Geometry check sheet. Reference: the model listing, model coordinates, mm. A direction names the side the tool comes from. Coordinates: 2 decimals unless noted, no trailing zeros. Write each loop counter-clockwise with the first axis right and the second up, starting at its lowest first coordinate (ties: lowest second). Pieces come first, ordered by that corner, then holes.
from build123d import *

# Parameters (mm, degrees)
SKETCH3_W           = 38.1
SKETCH3_H           = 38.1
BOSS_EXTRUDE2_DEPTH = 1.524
SKETCH4_W           = 16.002
SKETCH4_H           = 16.002
BOSS_EXTRUDE3_DEPTH = 7.112
SKETCH5_R           = 7.493
BOSS_EXTRUDE4_DEPTH = 12.192
BOSS_EXTRUDE6_DEPTH = 7.112


with BuildPart() as part:
    # Sketch3 → Boss-Extrude2 (new body)
    with BuildSketch(Plane(origin=(0, 0, 0), x_dir=(1, 0, 0), z_dir=(0, 1, 0))):
        Rectangle(SKETCH3_W, SKETCH3_H)
    extrude(amount=BOSS_EXTRUDE2_DEPTH)

    # Sketch4 → Boss-Extrude3 (add)
    with BuildSketch(Plane(origin=(0, 1.524, 0), x_dir=(1, 0, 0), z_dir=(0, 1, 0))):
        Rectangle(SKETCH4_W, SKETCH4_H)
    extrude(amount=BOSS_EXTRUDE3_DEPTH)

    # Sketch5 → Boss-Extrude4 (add)
    with BuildSketch(Plane(origin=(0, 8.636, 0), x_dir=(1, 0, 0), z_dir=(0, 1, 0))):
        with Locations(Location((0, 0, 0), (0, 0, 90))):
            Circle(SKETCH5_R)
    extrude(amount=BOSS_EXTRUDE4_DEPTH)

    # Sketch6 → Boss-Extrude6 (add)
    with BuildSketch(Plane(origin=(0, 8.636, 0), x_dir=(1, 0, 0), z_dir=(0, 1, 0))):
        with BuildLine():
            ThreePointArc((8.001, -0.71842049), (8.768319307, -1.717057132), (9.9695, -2.0955))
            ThreePointArc((9.9695, -2.0955), (11.45124226, -1.48174226), (12.065, 0))
            ThreePointArc((12.065, 0), (11.45124226, 1.48174226), (9.9695, 2.0955))
            ThreePointArc((9.9695, 2.0955), (8.768319307, 1.717057132), (8.001, 0.71842049))
            Line((8.001, 0.71842049), (8.001, -0.71842049))
        make_face()
        with BuildLine():
            ThreePointArc((8.001, 0.71842049), (7.874, 0), (8.001, -0.71842049))
            Line((8.001, -0.71842049), (8.001, 0.71842049))
        make_face()
        with BuildLine():
            Line((8.001, -2.0955), (9.9695, -2.0955))
            ThreePointArc((9.9695, -2.0955), (8.768319307, -1.717057132), (8.001, -0.71842049))
            Line((8.001, -0.71842049), (8.001, -2.0955))
        make_face()
        with BuildLine():
            Line((7.194020347, -2.0955), (8.001, -2.0955))
            Line((8.001, -2.0955), (8.001, -0.71842049))
            ThreePointArc((8.001, -0.71842049), (7.874, 0), (8.001, 0.71842049))
            Line((8.001, 0.71842049), (8.001, 2.0955))
            Line((8.001, 2.0955), (7.194020347, 2.0955))
            ThreePointArc((7.194020347, 2.0955), (7.417878519, 1.058360652), (7.493, 0))
            ThreePointArc((7.493, 0), (7.417878519, -1.058360652), (7.194020347, -2.0955))
        make_face()
        with BuildLine():
            ThreePointArc((8.001, 0.71842049), (8.768319307, 1.717057132), (9.9695, 2.0955))
            Line((9.9695, 2.0955), (8.001, 2.0955))
            Line((8.001, 2.0955), (8.001, 0.71842049))
        make_face()
        with BuildLine():
            Line((-7.194020347, -2.0955), (7.194020347, -2.0955))
            ThreePointArc((7.194020347, -2.0955), (7.417878519, -1.058360652), (7.493, 0))
            ThreePointArc((7.493, 0), (7.417878519, 1.058360652), (7.194020347, 2.0955))
            Line((7.194020347, 2.0955), (-7.194020347, 2.0955))
            ThreePointArc((-7.194020347, 2.0955), (-7.493, 0), (-7.194020347, -2.0955))
        make_face()
        with BuildLine():
            Line((-8.001, -2.0955), (-7.194020347, -2.0955))
            ThreePointArc((-7.194020347, -2.0955), (-7.493, 0), (-7.194020347, 2.0955))
            Line((-7.194020347, 2.0955), (-8.001, 2.0955))
            Line((-8.001, 2.0955), (-8.001, 0.55189456))
            ThreePointArc((-8.001, 0.55189456), (-7.945595412, 0.27841562), (-7.927017411, 0))
            ThreePointArc((-7.927017411, 0), (-7.945595412, -0.27841562), (-8.001, -0.55189456))
            Line((-8.001, -0.55189456), (-8.001, -2.0955))
        make_face()
        with BuildLine():
            ThreePointArc((-12.065, -0.468385659), (-11.328200782, -1.638997006), (-10.022517424, -2.0955))
            ThreePointArc((-10.022517424, -2.0955), (-8.750781359, -1.665475206), (-8.001, -0.55189456))
            Line((-8.001, -0.55189456), (-8.001, 0.55189456))
            ThreePointArc((-8.001, 0.55189456), (-8.75078136, 1.665475207), (-10.022517427, 2.0955))
            ThreePointArc((-10.022517427, 2.0955), (-11.328200783, 1.638997005), (-12.065, 0.468385659))
            Line((-12.065, 0.468385659), (-12.065, -0.468385659))
        make_face()
        with BuildLine():
            Line((-10.022517424, -2.0955), (-8.001, -2.0955))
            Line((-8.001, -2.0955), (-8.001, -0.55189456))
            ThreePointArc((-8.001, -0.55189456), (-8.750781359, -1.665475206), (-10.022517424, -2.0955))
        make_face()
        with BuildLine():
            Line((-8.001, 0.55189456), (-8.001, -0.55189456))
            ThreePointArc((-8.001, -0.55189456), (-7.945595412, -0.27841562), (-7.927017411, 0))
            ThreePointArc((-7.927017411, 0), (-7.945595412, 0.27841562), (-8.001, 0.55189456))
        make_face()
        with BuildLine():
            Line((-8.001, 0.55189456), (-8.001, 2.0955))
            Line((-8.001, 2.0955), (-10.022517427, 2.0955))
            ThreePointArc((-10.022517427, 2.0955), (-8.75078136, 1.665475207), (-8.001, 0.55189456))
        make_face()
    extrude(amount=-BOSS_EXTRUDE6_DEPTH)

    # Sketch8 → Cut-Revolve2 (revolve, cut)
    with BuildSketch(Plane.XY, mode=Mode.PRIVATE) as cut_revolve2_sk:
        with BuildLine():
            ThreePointArc((-3.683327211, 18.4271959), (-2.28773348, 20.259113148), (-0.056148749, 20.828))
            ThreePointArc((-0.056148749, 20.828), (-3.774574374, 21.391967579), (-7.493, 20.828))
            ThreePointArc((-7.493, 20.828), (-5.455602523, 19.837950118), (-3.683327211, 18.4271959))
        make_face()
    revolve(cut_revolve2_sk.sketch.rotate(Axis((0, 0, 0), (0, 1, 0)), 270), axis=Axis((0, 0, 0), (0, 1, 0)), mode=Mode.SUBTRACT)


solid = part.part
1. Sectioned sample at A-A, the plane y = 10. Record the boundary of the cut face in (x, z).
Computed values:
outline: circle Ø14.99 at (0, 0)
2. Thickness scan on line 1 along Y through (x, z) = (-2.5, -11.5); line 2 along Z through (x, y) = (1, 2.25). Record the ranges inside material, lowest first.
Computed values:
line 1: y = 0 to 1.52
line 2: z = -8 to 8
3. Gauge pin test, flat ends, axial feed: pin 1 Ø5 at (x, y) = (-8.5, 10.5) entering from +Z; pin 2 Ø3 at (y, z) = (7, -5.5) entering from +X; pin 3 Ø4 at (x, z) = (11, -10) entering from +Y. Record the tip position at first contact, or that the pin passes through.
Computed values:
pin 1: stops at z = 8
pin 2: stops at x = 8
pin 3: stops at y = 1.52
4. Access from +Z, -Z, +X, -X, +Y, -Y to the whole of each face (thin tool, end or side, straight path). Record for faces 1 (the cylindrical face through (-11.34, 5.13, 1.63)), 2 (the flat face through (7.1, 8.636, -3)), 3 (the flat face through (8.001, 5, 5)), 4 (the flat face through (-8.001, 5, -5)), 5 (the flat face through (8.001, 5, -5)).
Computed values:
face 1: +Z, -X, +Y
face 2: +Y
face 3: +Z, +X, +Y
face 4: -Z, -X, +Y
face 5: -Z, +X, +Y
5. Sectioned sample at B-B, the plane z = 13.5. Record the boundary of the cut face in (x, y), and give its area (3 significant figures).
Computed values:
outline: (-19.05, 0) - (19.05, 0) - (19.05, 1.52) - (-19.05, 1.52) - close
area: 58.1 mm2
